Model file for the job. Use its own axes, mm. A direction names the side the tool comes from. Round coordinates to 2 decimals unless told otherwise and drop trailing zeros. Write each loop counter-clockwise with the first axis right and the second up, starting at its lowest first coordinate (ties: lowest second). Pieces come first, ordered by that corner, then holes.
```python
from build123d import *

# Parameters (mm, degrees)
SKETCH1_R           = 3
BOSS_EXTRUDE1_DEPTH = 90
SKETCH2_R           = 5.8
BOSS_EXTRUDE2_DEPTH = 4.3
FILLET1_R           = 1


with BuildPart() as part:
    # Sketch1 → Boss-Extrude1 (new body)
    with BuildSketch(Plane(origin=(0, 0, 0), x_dir=(1, 0, 0), z_dir=(0, 1, 0))):
        with Locations(Location((0, 0, 0), (0, 0, 270))):  # turned: the seam where the file's is
            Circle(SKETCH1_R)
    extrude(amount=BOSS_EXTRUDE1_DEPTH)

    # Sketch2 → Boss-Extrude2 (add)
    with BuildSketch(Plane(origin=(0, 90, 0), x_dir=(1, 0, 0), z_dir=(0, 1, 0))):
        with Locations(Location((0, 0, 0), (0, 0, 270))):  # turned: the seam where the file's is
            Circle(SKETCH2_R)
    extrude(amount=BOSS_EXTRUDE2_DEPTH)

    # Fillet1
    fillet1_edges = [part.edges().sort_by_distance(p)[0] for p in [
        (0, 90, -5.8),
        (0, 94.3, -5.8),
    ]]
    fillet(fillet1_edges, radius=FILLET1_R)


solid = part.part
```
1) Cut at B-B on x = 0. List the corners of the cut face in (y, z).
2) Cut at C-C on y = 27.5. List the corners of the cut face in (x, z).
3) Flat gauge pins, fed straight in: pin 1 Ø1 at (x, y) = (-2.5, 44) entering from +Z; pin 2 Ø6 at (x, y) = (0, 48.5) entering from +Z; pin 3 Ø1.5 at (x, y) = (-3, 16.5) entering from -Z. Where does each tip first touch, or does it go through?
4) Wall check: probe 1 along Y at (x, z) = (-3, 1.5); probe 2 along X at (y, z) = (50, 0.25); probe 3 along Z at (x, y) = (0.75, 76.5). Give the ranges that are in metal, low to high.
5) Which spindle directions (+Z, -Z, +X, -X, +Y, -Y) get a long thin tool onto all of the face, cutting with end or side? Do faces 1 (the face through (-3, 90, 1)), 2 (the face through (0, 0, 0)). Say none if no direction does.
6) Cut at A-A on z = 0. List the corners of the cut face in (x, y).
Result sheet:
1. outline: (0, -3) - (90, -3) - (90, -4.8) arc R1 ccw to (91, -5.8) - (93.3, -5.8) arc R1 ccw to (94.3, -4.8) - (94.3, 4.8) arc R1 ccw to (93.3, 5.8) - (91, 5.8) arc R1 ccw to (90, 4.8) - (90, 3) - (0, 3) - close
2. outline: circle Ø6 at (0, 0)
3. pin 1: stops at z = 2.24
3. pin 2: stops at z = 3
3. pin 3: stops at z = -1.98
4. probe 1: y = 90 to 94.3
4. probe 2: x = -2.99 to 2.99
4. probe 3: z = -2.9 to 2.9
5. face 1: -Y
5. face 2: +Z, -Z, +X, -X, -Y
6. outline: (-5.8, 91) arc R1 ccw to (-4.8, 90) - (-3, 90) - (-3, 0) - (3, 0) - (3, 90) - (4.8, 90) arc R1 ccw to (5.8, 91) - (5.8, 93.3) arc R1 ccw to (4.8, 94.3) - (-4.8, 94.3) arc R1 ccw to (-5.8, 93.3) - close
